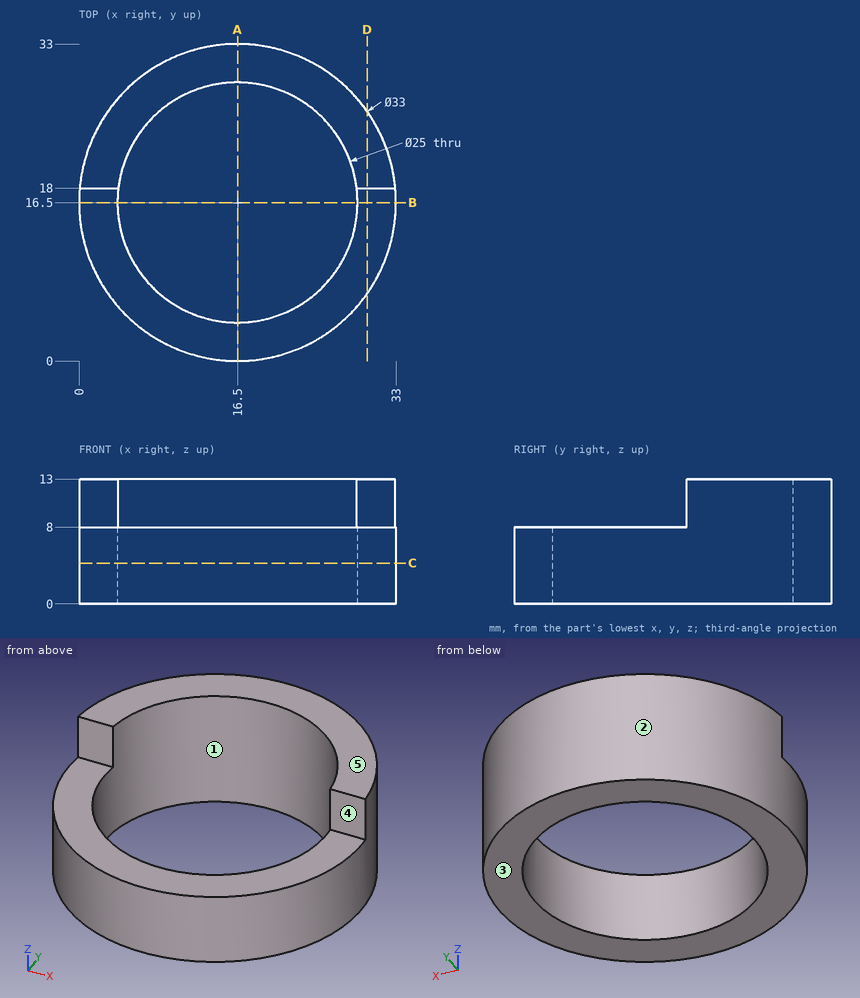
Check sheet for the drawn part. Datum: minimum x, y, z corner. Units: mm. A direction names the side the tool comes from. Give positions to 0.01 mm unless a question says otherwise; leave off trailing zeros. Write each loop counter-clockwise with the first axis right and the second up, starting at its lowest first coordinate (ties: lowest second). Pieces come first, ordered by that corner, then holes. Notation, with made-up numbers: M 76.25,85.25 L 110.25,85.25 A9 cw 110.25,92.25 Z; hole C 68.25,42.25 d5. An arc over 180 degrees is marked long. One line per question, with ' | ' between items.
1. Set-up check for the marked faces 4 and 5: record each of +Z, -Z, +X, -X, +Y, -Y from which the full face is reachable in a straight line by a thin tool's end or side.
Ans:
face 4: +Z, +X, -X, -Y | face 5: +Z, +X, -X, +Y, -Y
2. Cross-section at D-D (x = 30). Enter the section's corners in (y, z).
Ans:
outline: M 7.01,0 L 25.99,0 L 25.99,13 L 18,13 L 18,8 L 7.01,8 Z
3. Gauge pin test, flat ends, axial feed: pin 1 (3 mm diameter, centred on x = 25.5, z = 11.5, fed in from -Y); pin 2 (1.5 mm diameter, centred on y = 19, z = 1.5, fed in from +X); pin 3 (2 mm diameter, centred on x = 1.5, z = 11.5, fed in from -Y). Record the tip position at first contact, or that the pin passes through.
Ans:
pin 1: y = 23.28 | pin 2: x = 32.91 | pin 3: y = 18
4. Cross-section at C-C (z = 4.25). Enter the section's corners in (x, y), plus the area to 3 significant figures.
Ans:
outline: C 16.5,16.5 d33; hole C 16.5,16.5 d25 | area: 364 mm2
5. Cross-section at A-A (x = 16.5). Enter the section's corners in (y, z).
Ans:
outline: M 0,0 L 4,0 L 4,8 L 0,8 Z; M 29,0 L 33,0 L 33,13 L 29,13 Z
6. Mould release check, pull along Y, two halves, no side actions. Record for the marked faces 1, 2 and 3: released by +Y, released by -Y, zero draft, split by the parting line, or undercut.
Ans:
face 1: undercut | face 2: split by the parting line | face 3: zero draft
7. Cross-section at B-B (y = 16.5). Enter the section's corners in (x, z).
Ans:
outline: M 0,0 L 4,0 L 4,8 L 0,8 Z; M 29,0 L 33,0 L 33,8 L 29,8 Z
8. Scan lines: line 1 along Y through (x, z) = (15, 0.5); line 2 along Y through (x, z) = (16.5, 7.5). Record each from-to range of solid material in increasing order. Write a range as from..to.
Ans:
line 1: 0.07..4.09, 28.91..32.93 | line 2: 0..4, 29..33
